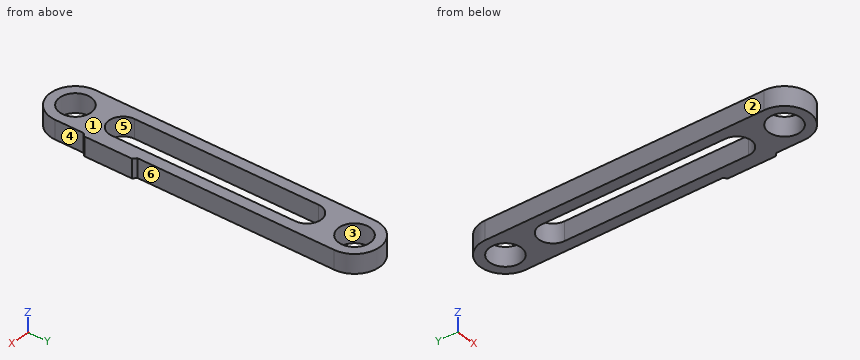
from build123d import *

# Parameters (mm, degrees)
SKETCH_1_R          = 5
EXTRUDE_1_DEPTH     = 6
CUT_EXTRUDE_1_DEPTH = 10
SKETCH_3_W          = 1
SKETCH_3_H          = 15
EXTRUDE_2_DEPTH     = 6
CHAMFER_1_SIZE      = 1


with BuildPart() as part:
    # 草图1 → 凸台-拉伸1 (new body)
    with BuildSketch(Plane.XY):
        with BuildLine():
            Line((-8, 0), (-8, 88))
            ThreePointArc((-8, 88), (0, 96), (8, 88))
            Line((8, 88), (8, 0))
            ThreePointArc((8, 0), (0, -8), (-8, 0))
        make_face()
        with Locations((0, 88)):
            Circle(SKETCH_1_R, mode=Mode.SUBTRACT)
        Circle(SKETCH_1_R, mode=Mode.SUBTRACT)
    extrude(amount=EXTRUDE_1_DEPTH)

    # 草图2 → 切除-拉伸1 (cut)
    with BuildSketch(Plane(origin=(0, 0, 0), x_dir=(-1, 0, 0), z_dir=(0, 0, -1))):
        with BuildLine():
            Line((4.5, 73), (4.5, 15))
            ThreePointArc((4.5, 15), (0, 10.5), (-4.5, 15))
            Line((-4.5, 15), (-4.5, 73))
            ThreePointArc((-4.5, 73), (0, 77.5), (4.5, 73))
        make_face()
    extrude(amount=-CUT_EXTRUDE_1_DEPTH, mode=Mode.SUBTRACT)

    # 草图3 → 凸台-拉伸2 (add)
    with BuildSketch(Plane.XY.offset(6)):
        with Locations((8.5, 17.5)):
            Rectangle(SKETCH_3_W, SKETCH_3_H)
    extrude(amount=-EXTRUDE_2_DEPTH)

    # 倒角1
    chamfer_1_edges = [part.edges().sort_by_distance(p)[0] for p in [
        (8, 10, 3),
        (8, 25, 3),
    ]]
    chamfer(chamfer_1_edges, length=CHAMFER_1_SIZE - 0.0001)  # a hair under: the kernel refuses the full size


solid = part.part
Part model, mm, in its own coordinate system. Face numbers are marked on the shaded views. A direction names the side the tool comes from. Coordinates: 2 decimals unless noted, no trailing zeros. Order: outer loops, then holes, each group sorted by start corner. A loop starts at its lowest first (then second) coordinate and runs counter-clockwise, first axis right, second up. Notation, with made-up numbers: M -15.75,69.5 L 32.25,69.5 A26 cw 32.25,101.5 Z; hole C 20.25,11 d8. An arc over 180 degrees is marked long. One line per question, with ' | ' between items.
Q1. Drill centre lines: line 1 (Y direction, x = 0, z = 3.1); line 2 (X direction, y = 69, z = 1.1); line 3 (Y direction, x = 3.5, z = 1.8). Where is each one in solid material? Low to high.
A:
line 1: y = -8 to -5, 5 to 10.5, 77.5 to 83, 93 to 96 | line 2: x = -8 to -4.5, 4.5 to 8 | line 3: y = -7.19 to -3.57, 3.57 to 12.17, 75.83 to 84.43, 91.57 to 95.19
Q2. Pin check, flat tips, straight feed: P1, Ø3, axis at x = 2, y = 46, coming from the -Z side; P2, Ø3, axis at y = 39, z = 3.5, coming from the +X side; P3, Ø1, axis at x = -2.5, z = 4, coming from the +Y side. Stop position of each tip, or through.
A:
P1: passes through | P2: stops at x = 8 | P3: stops at y = 95.75
Q3. Slice it at D-D (y = 72). Give the cut face in (x, z).
A:
outline: M -8,0 L -4.5,0 L -4.5,6 L -8,6 Z; M 4.5,0 L 8,0 L 8,6 L 4.5,6 Z
Q4. Slice it at A-A (x = 0). Give the cut face in (y, z).
A:
outline: M -8,0 L -5,0 L -5,6 L -8,6 Z; M 5,0 L 10.5,0 L 10.5,6 L 5,6 Z; M 77.5,0 L 83,0 L 83,6 L 77.5,6 Z; M 93,0 L 96,0 L 96,6 L 93,6 Z
Q5. 3-axis set-ups, long thin cutter, end or side, ignore diameter. For the marked faces 4, 5 and 6: which of +Z, -Z, +X, -X, +Y, -Y reach the whole face in a straight line?
A:
face 4: +Z, -Z, +X, -Y | face 5: +Z, -Z | face 6: +Z, -Z, +X, +Y
Q6. Two-plate mould, pull along X, no slides. Class the marked faces 1, 2 and 3: +X half, -X half, draft (parallel to the pull), parting line (faces both ways), or undercut.
A:
face 1: draft | face 2: -X half | face 3: undercut
Q7. Slice it at C-C (z = 4.25). Count the separate pieces of the cut face and the enclosed holes in it, and give its area (3 significant figures).
A:
separate pieces: 1 | enclosed holes: 3 | area: 882 mm^2
Q8. Slice it at B-B (y = 16.5). Give the cut face in (x, z), and give its area (3 significant figures).
A:
outline: M -8,0 L -4.5,0 L -4.5,6 L -8,6 Z; M 4.5,0 L 9,0 L 9,6 L 4.5,6 Z | area: 48.0 mm^2
